```python
from build123d import *

# Parameters (mm, degrees)
SKIZZE4_W          = 0.25
SKIZZE4_H          = 1
TOOLFACE_ANGLE     = 60
KREISMUSTER1_COUNT = 3


with BuildPart() as part:
    # Skizze3 → Body (revolve)
    with BuildSketch(Plane.XY):
        with BuildLine():
            Line((1, 0.8), (2.75, 0.8))
            Line((2.75, 0.8), (2.75, -2.55))
            Line((2.75, -2.55), (2.1, -2.55))
            Line((2.1, -2.55), (1.8, -2.25))
            ThreePointArc((1.8, -2.25), (0.91241438, -2.474486277), (0, -2.55))
            Line((0, -2.55), (0, 0.525))
            ThreePointArc((0, 0.525), (0.316474723, 0.499842016), (0.625, 0.425))
            Line((0.625, 0.425), (1, 0.8))
        make_face()
    revolve(axis=Axis((0, 0, 0), (0, -1, 0)))

    # Skizze4 → Thread (revolve)
    with BuildSketch(Plane.XY):
        with Locations((2.875, -0.7)):
            Rectangle(SKIZZE4_W, SKIZZE4_H)
    revolve(axis=Axis((0, 0, 0), (0, 1, 0)))

    # Skizze5 → Toolface (revolve, cut)
    with BuildSketch(Plane(origin=(0, 0, 0), x_dir=(0, 0, -1), z_dir=(1, 0, 0))):
        Polygon((2.75, 0.8), (2.75, 0.35), (2.3, 0.8), align=None)
    toolface = revolve(axis=Axis((0, 0, 0), (0, -1, 0)), revolution_arc=TOOLFACE_ANGLE, mode=Mode.SUBTRACT)

    # Kreismuster1: Toolface ×3 about axis
    kreismuster1_axis = Axis((0, 0, 0), (0, 1, 0))
    for i in range(1, KREISMUSTER1_COUNT):
        add(toolface.rotate(kreismuster1_axis, i * 360 / KREISMUSTER1_COUNT), mode=Mode.SUBTRACT)


solid = part.part
```
The model under review builds one solid part; all positions refer to its coordinate system, in mm. A direction names the side the tool comes from. Coordinates: 2 decimals unless noted, no trailing zeros. Write each loop counter-clockwise with the first axis right and the second up, starting at its lowest first coordinate (ties: lowest second). Pieces come first, ordered by that corner, then holes. Notation, with made-up numbers: (87.5, -10.5) - (110.5, -10.5) arc R13 cw to (110.5, 6.5) - close; hole circle Ø9 at (84, -27.75). An arc over 180 degrees is marked (long way). Answer in a Markdown table with one row per item. Add a question column.
Q1. Consider section C-C on y = -1. Give the boundary of the cut face in (x, z), then the cut area to 3 significant figures.
Q2. Consider section A-A on z = 0. Give the boundary of the cut face in (x, y) (3 decimals), then the cut area to 3 significant figures.
Q3. Clearance check with a flat-ended pin moving along its axis: pin 1 (1.5 mm diameter, centred on x = 1, y = -1.5, fed in from -Z). State where the tip first meets the part, or that it passes through.
Q4. To check wall thickness, follow line 1 along Y through (x, z) = (-1.2, 2.65); line 2 along Y through (x, z) = (-1.3, -1); line 3 along Z through (x, y) = (-0.25, 0.6). State the ranges of each line that lie inside material, in increasing order. Write a range as from..to.
Q5. Consider section B-B on y = -1.9. Give the boundary of the cut face in (x, z), then the cut area to 3 significant figures.
Q6. For faces 1 (the face through (-0.596, -1.884, -2.685)), 2 (the face through (2.62, 0.29, 0.83)), 3 (the face through (-3, -1, 0)), list the 3-axis set-ups (+Z, -Z, +X, -X, +Y, -Y) from which the entire face can be reached by the end or side of a thin tool; tool diameter is ignored.
Answers below:
| question | item | result |
|---|---|---|
| 1 | outline | circle Ø6 at (0, 0) |
| 1 | area | 28.3 mm² |
| 2 | outline | (-3, -1.2) - (-2.75, -1.2) - (-2.75, -2.55) - (-2.1, -2.55) - (-1.8, -2.25) arc R5.55 ccw to (1.8, -2.25) - (2.1, -2.55) - (2.75, -2.55) - (2.75, -1.2) - (3, -1.2) - (3, -0.2) - (2.75, -0.2) - (2.75, 0.8) - (1, 0.8) - (0.625, 0.425) arc R2.003 ccw to (-0.625, 0.425) - (-1, 0.8) - (-2.3, 0.8) - (-2.75, 0.35) - (-2.75, -0.2) - (-3, -0.2) - close |
| 2 | area | 17.9 mm² |
| 3 | pin 1 | z = -2.98 |
| 4 | line 1 | -1.2..-0.2 |
| 4 | line 2 | -2.3..0.8 |
| 4 | line 3 | -2.74..-0.76, 0.76..2.74 |
| 5 | outline | circle Ø5.5 at (0, 0) |
| 5 | area | 23.8 mm² |
| 6 | face 1 | -Y |
| 6 | face 2 | +Y |
| 6 | face 3 | +Y, -Y |
